Design review of the part built by this model. Coordinates are the model's own, in mm. Face numbers are marked on the shaded views. A direction names the side the tool comes from. Give positions to 0.01 mm unless a question says otherwise; leave off trailing zeros. Write each loop counter-clockwise with the first axis right and the second up, starting at its lowest first coordinate (ties: lowest second). Pieces come first, ordered by that corner, then holes. Notation, with made-up numbers: M 56.25,42 L 112.25,42 A27 ccw 112.25,63 Z; hole C 44.5,22 d1. An arc over 180 degrees is marked long. One line per item, written item: value. Start each with the question number.
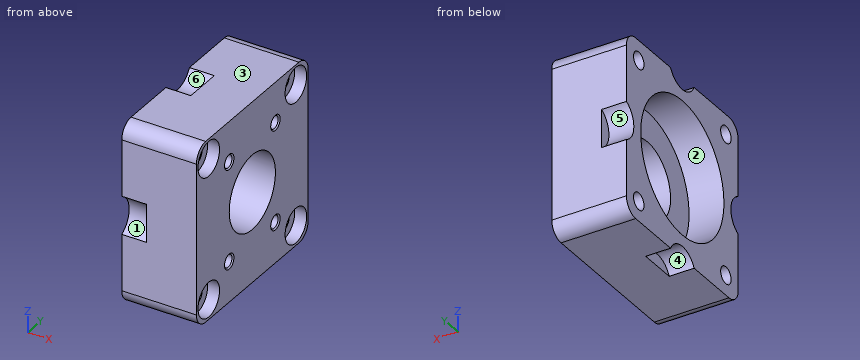
```python
from build123d import *

# Parameters (mm, degrees)
SKETCH1_W                                        = 36.284271248
SKETCH1_H                                        = 36.284271248
BOSS_EXTRUDE1_DEPTH                              = 15
CUT_EXTRUDE1_DEPTH                               = 7
CUT_EXTRUDE1_DEPTH_BACK                          = 30.719928835
SKETCH1_4_R                                      = 13.5
SKETCH1_4_R_2                                    = 7.5
CUT_EXTRUDE2_DEPTH                               = 30.719928835
CUT_EXTRUDE2_DEPTH_BACK                          = 30.719928835
SKETCH1_5_R                                      = 7.5
FILLET1_R                                        = 3
CBORE_FOR_M3_PAN_HEAD_MACHINE_SCREW1_D           = 3.4
CBORE_FOR_M3_PAN_HEAD_MACHINE_SCREW1_CBORE_D     = 7
CBORE_FOR_M3_PAN_HEAD_MACHINE_SCREW1_CBORE_DEPTH = 2.4
SKETCH1_6_R                                      = 4.25
CUT_EXTRUDE3_DEPTH                               = 5


# Read off the part's stored shape, not the designer's step: M3x0.5 Tapped Hole1
with BuildPart() as part:
    # Sketch1 → Boss-Extrude1 (new body)
    with BuildSketch(Plane(origin=(0, 0, 0), x_dir=(0, 0, -1), z_dir=(1, 0, 0))):
        Rectangle(SKETCH1_W, SKETCH1_H)
    extrude(amount=BOSS_EXTRUDE1_DEPTH)

    # Sketch1<4> → Cut-Extrude1 (cut, two sides: drawn at the far end of the back side and taken through both)
    with BuildSketch(Plane(origin=(0, 0, 0), x_dir=(0, 0, -1), z_dir=(1, 0, 0)).offset(-CUT_EXTRUDE1_DEPTH_BACK)):
        with Locations(Location((0, 0, 0), (0, 0, 180))):
            Circle(SKETCH1_4_R)
        with Locations(Location((0, 0, 0), (0, 0, 180))):
            Circle(SKETCH1_4_R_2, mode=Mode.SUBTRACT)
    extrude(amount=CUT_EXTRUDE1_DEPTH + CUT_EXTRUDE1_DEPTH_BACK, mode=Mode.SUBTRACT)

    # Sketch1<5> → Cut-Extrude2 (cut, two sides: drawn at the far end of the back side and taken through both)
    with BuildSketch(Plane(origin=(0, 0, 0), x_dir=(0, 0, -1), z_dir=(1, 0, 0)).offset(-CUT_EXTRUDE2_DEPTH_BACK)):
        Circle(SKETCH1_5_R)
    extrude(amount=CUT_EXTRUDE2_DEPTH + CUT_EXTRUDE2_DEPTH_BACK, mode=Mode.SUBTRACT)

    # M3x0.5 Tapped Hole1 outline → M3x0.5 Tapped Hole1 (revolve, cut)
    with BuildSketch(Plane(origin=(0, -7.5, -10), x_dir=(0, 1, 0), z_dir=(0, 0, -1))):
        Polygon((0, 15), (0, 9.248924226), (1.25, 10), (1.25, 14.769247601), (1.525, 15), align=None)
    revolve(axis=Axis((0, -7.5, -10), (1, 0, 0)), mode=Mode.SUBTRACT)

    # M3x0.5 Tapped Hole1 2 outline → M3x0.5 Tapped Hole1 2 (revolve, cut)
    with BuildSketch(Plane(origin=(0, 7.5, 10), x_dir=(0, 1, 0), z_dir=(0, 0, -1))):
        Polygon((0, 15), (0, 9.248924226), (1.25, 10), (1.25, 14.769247601), (1.525, 15), align=None)
    revolve(axis=Axis((0, 7.5, 10), (1, 0, 0)), mode=Mode.SUBTRACT)

    # M3x0.5 Tapped Hole1 3 outline → M3x0.5 Tapped Hole1 3 (revolve, cut)
    with BuildSketch(Plane(origin=(0, -7.5, 10), x_dir=(0, 1, 0), z_dir=(0, 0, -1))):
        Polygon((0, 15), (0, 9.248924226), (1.25, 10), (1.25, 14.769247601), (1.525, 15), align=None)
    revolve(axis=Axis((0, -7.5, 10), (1, 0, 0)), mode=Mode.SUBTRACT)

    # M3x0.5 Tapped Hole1 4 outline → M3x0.5 Tapped Hole1 4 (revolve, cut)
    with BuildSketch(Plane(origin=(0, 7.5, -10), x_dir=(0, 1, 0), z_dir=(0, 0, -1))):
        Polygon((0, 15), (0, 9.248924226), (1.25, 10), (1.25, 14.769247601), (1.525, 15), align=None)
    revolve(axis=Axis((0, 7.5, -10), (1, 0, 0)), mode=Mode.SUBTRACT)

    # Fillet1
    fillet1_edges = [part.edges().sort_by_distance(p)[0] for p in [
        (7.5, -18.142135624, 18.142135624),
        (7.5, -18.142135624, -18.142135624),
        (7.5, 18.142135624, -18.142135624),
        (7.5, 18.142135624, 18.142135624),
    ]]
    fillet(fillet1_edges, radius=FILLET1_R)

    # CBORE for M3 Pan Head Machine Screw1 (through all)
    with Locations(Plane(origin=(15, 0, 0), x_dir=(0, 0, -1), z_dir=(1, 0, 0))):
        with Locations((14.142135624, 14.142135624), (-14.142135624, 14.142135624), (-14.142135624, -14.142135624), (14.142135624, -14.142135624)):
            CounterBoreHole(CBORE_FOR_M3_PAN_HEAD_MACHINE_SCREW1_D / 2, CBORE_FOR_M3_PAN_HEAD_MACHINE_SCREW1_CBORE_D / 2, CBORE_FOR_M3_PAN_HEAD_MACHINE_SCREW1_CBORE_DEPTH)

    # Sketch1<6> → Cut-Extrude3 (cut)
    with BuildSketch(Plane(origin=(0, 0, 0), x_dir=(0, 0, -1), z_dir=(1, 0, 0))):
        with Locations((0, 20)):
            Circle(SKETCH1_6_R)
        with Locations((0, -20)):
            Circle(SKETCH1_6_R)
        with Locations((20, 0)):
            Circle(SKETCH1_6_R)
        with Locations((-20, 0)):
            Circle(SKETCH1_6_R)
    extrude(amount=CUT_EXTRUDE3_DEPTH, mode=Mode.SUBTRACT)


solid = part.part
```
Q1. Machinability: for the marked faces 1, 2 and 3, which of the approach directions +Z, -Z, +X, -X, +Y, -Y give a long, thin tool a straight path to every point of the face, cutting with its end or side? Answer none if there is none.
Q2. Take a section at C-C, the plane x = 4.25. Give the boundary of the cut face in (y, z).
Q3. Take a section at D-D, the plane x = 13.75. State how many separate pieces and enclosed holes the cut face has, then the cut area to 3 significant figures.
Q4. The part is to be moulded in two halves that separate along Z. For the marked faces 4, 5 and 6, say which applies: pulls with the +Z half, pulls with the -Z half, needs draft (parallel to the pull), parting line crosses it, or undercut.
Q5. For P1, Ø1.9, axis at y = 1.5, z = 17.5, coming from the -X side; P2, Ø2, axis at y = 7.5, z = -10, coming from the +X side; P3, Ø4, axis at y = 14.14, z = 14.14, coming from the +X side, all flat-tipped, find the tip position at first contact; note any pin that passes through.
Q6. Take a section at A-A, the plane z = 0. Give the boundary of the cut face in (x, y), then the cut area to 3 significant figures.
Q7. Wall thickness on line 1 (Y direction, x = 6.25, z = -14); line 2 (Z direction, x = 13.5, y = 16.5); line 3 (X direction, y = 1.5, z = -7.5): over which ranges is each line inside the solid? List them lowest first. Write a range as from..to.
Results list:
1. face 1: -X, -Y
1. face 2: -X
1. face 3: +Z, +X, -X, +Y, -Y
2. outline: M -18.14,-15.14 A3 ccw -15.14,-18.14 L -3.82,-18.14 A4.25 cw 3.82,-18.14 L 15.14,-18.14 A3 ccw 18.14,-15.14 L 18.14,-3.82 A4.25 cw 18.14,3.82 L 18.14,15.14 A3 ccw 15.14,18.14 L 3.82,18.14 A4.25 cw -3.82,18.14 L -15.14,18.14 A3 ccw -18.14,15.14 L -18.14,3.82 A4.25 cw -18.14,-3.82 Z; hole C -14.14,-14.14 d3.4; hole C -14.14,14.14 d3.4; hole C 0,0 d27; hole C 14.14,-14.14 d3.4; hole C 14.14,14.14 d3.4
3. separate pieces: 1
3. enclosed holes: 9
3. area: 959 mm^2
4. face 4: pulls with the -Z half
4. face 5: undercut
4. face 6: pulls with the +Z half
5. P1: stops at x = 5
5. P2: stops at x = 9.85
5. P3: stops at x = 12.6
6. outline: M 0,-15.75 L 5,-15.75 L 5,-18.14 L 15,-18.14 L 15,-7.5 L 7,-7.5 L 7,-13.5 L 0,-13.5 Z; M 0,13.5 L 7,13.5 L 7,7.5 L 15,7.5 L 15,18.14 L 5,18.14 L 5,15.75 L 0,15.75 Z
6. area: 211 mm^2
7. line 1: y = -18.14..-15.84, -12.45..12.45, 15.84..18.14
7. line 2: z = -17.82..-16.73, -11.56..11.56, 16.73..17.82
7. line 3: x = 7..15
